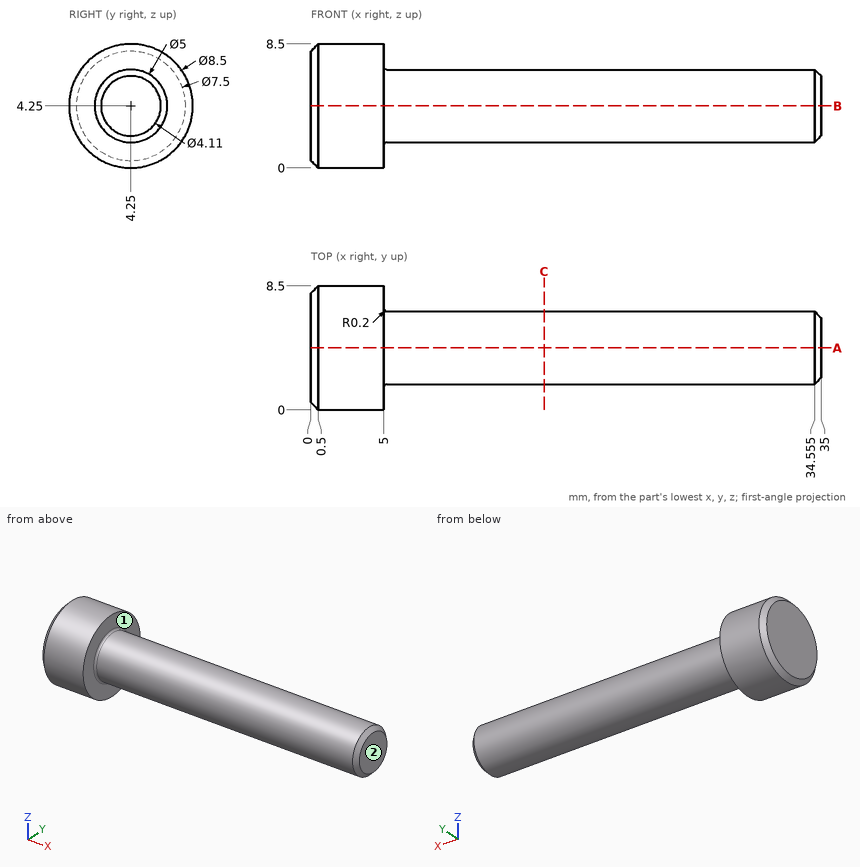
The figure shows three views and two pictorial views of one solid part (mm, origin at its lowest corner). Answer the questions. A direction names the side the tool comes from. Round coordinates to 2 decimals unless told otherwise and drop trailing zeros. Write each loop counter-clockwise with the first axis right and the second up, starting at its lowest first coordinate (ties: lowest second). Pieces come first, ordered by that corner, then holes. Notation, with made-up numbers: (30.5, 16.5) -> (76.5, 16.5) arc R34 ccw to (76.5, 47.5) -> close; hole circle Ø10 at (50.5, -39). An arc over 180 degrees is marked (long way). Answer as a JSON object with one key per item and string values. Group by question number.
Q1. Each of these flat-tipped pins is pushed along its axis until it touches: pin 1 Ø3 at (y, z) = (7, 4.5) entering from -X; pin 2 Ø1.5 at (x, y) = (11.5, 5.5) entering from +Z; pin 3 Ø3 at (x, y) = (21.5, 2) entering from -Z; pin 4 Ø5 at (x, y) = (10, 5.5) entering from -Z. Where does it stop, or does it pass through?
Q2. Straight lines are drawn through the part: line 1 along X through (y, z) = (1.5, 6.25); line 2 along Y through (x, z) = (3.5, 7); line 3 along Y through (x, z) = (26.5, 6.5). For each, find the intervals that lie inside material, in ascending order.
Q3. Section A-A (y = 4.25) is taken. Write down the section's boundary in (x, z) (3 decimals).
Q4. Which of the six approach directions +Z, -Z, +X, -X, +Y, -Y give full straight-line access (tool end or side, diameter ignored) to the marked faces 1 and 2?
Q5. Section C-C (x = 16) is taken. Write down the section's boundary in (y, z), plus the area to 3 significant figures.
Check values:
{
 "1": {"pin 1": "x = 0", "pin 2": "z = 6.7", "pin 3": "z = 1.87", "pin 4": "z = 1.75"},
 "2": {"line 1": "0 to 5", "line 2": "1.01 to 7.49", "line 3": "3.16 to 5.34"},
 "3": {"outline": "(0, 0.5) -> (0.5, 0) -> (5, 0) -> (5, 1.55) arc R0.2 cw to (5.2, 1.75) -> (34.555, 1.75) -> (35, 2.195) -> (35, 6.305) -> (34.555, 6.75) -> (5.2, 6.75) arc R0.2 cw to (5, 6.95) -> (5, 8.5) -> (0.5, 8.5) -> (0, 8) -> close"},
 "4": {"face 1": "+X", "face 2": "+Z, -Z, +X, +Y, -Y"},
 "5": {"outline": "circle Ø5 at (4.25, 4.25)", "area": "19.6 mm^2"}
}
